from build123d import *

# Parameters (mm, degrees)
BASE_DEPTH                                          = 5
BASE_FILLET_R                                       = 1.65
HOOK_BASE_REACH                                     = 15.601
HOOK_BASE_END_RADIUS                                = 1.65
CBORE_FOR_M2_HEX_SOCKET_HEAD_CAP_SCREW1_D           = 2.4
CBORE_FOR_M2_HEX_SOCKET_HEAD_CAP_SCREW1_DEPTH       = 7.25
CBORE_FOR_M2_HEX_SOCKET_HEAD_CAP_SCREW1_CBORE_D     = 4.4
CBORE_FOR_M2_HEX_SOCKET_HEAD_CAP_SCREW1_CBORE_DEPTH = 2.4
CBORE_FOR_M2_HEX_SOCKET_HEAD_CAP_SCREW1_TIP         = 0.7210327428330723
SKETCH16_W                                          = 5.000000000000002
SKETCH16_H                                          = 1.65
SKETCH6_W                                           = 1.1499999999999981
SKETCH6_H                                           = 2.0000000000000004
CUT_EXTRUDE4_DEPTH                                  = 7.85
CIRPATTERN1_COUNT                                   = 2
FILLET1_R                                           = 1.65


with BuildPart() as part:
    # Sketch1 → Base (new body)
    # profile 1 of 2: a face of its own
    with BuildSketch(Plane(origin=(0, 0, 0), x_dir=(0, 1, 0), z_dir=(0, 0, 1))):
        Polygon((12.000000000000002, 4), (12.000000000000004, -3.9999999999999947), (-12, -4), (-12.000000000000002, 4), align=None)
        Polygon((-10, 2.35), (10, 2.35), (10, -2.35), (-9.999999999999998, -2.35), align=None, mode=Mode.SUBTRACT)
    # profile 2 of 2: a face of its own
    with BuildSketch(Plane(origin=(0, 0, 0), x_dir=(0, 1, 0), z_dir=(0, 0, 1))):
        Polygon((10, 2.35), (10, -2.35), (-9.999999999999998, -2.35), (-10, 2.35), align=None)
    extrude(amount=BASE_DEPTH)

    # Base-Fillet
    base_fillet_edges = [part.edges().sort_by_distance(p)[0] for p in [
        (-4, 0, 5),
        (3.9999999999999973, 1.78e-15, 5),
    ]]
    fillet(base_fillet_edges, radius=BASE_FILLET_R)

    # Hook Base: up to this cylinder (the profile starts outside it)
    hook_base_end = Plane(origin=(-2.35, 9.5, 3.35), z_dir=(0, 1, 0)) * Cylinder(HOOK_BASE_END_RADIUS, 35.502, mode=Mode.PRIVATE)
    # Sketch - Hook Base → Hook Base (add, up to the surface)
    with BuildSketch(Plane.XY.offset(5), mode=Mode.PRIVATE) as hook_base_sk1:
        Polygon((-4, 12.000000000000002), (-2.850000000000002, 12.000000000000004), (-2.850000000000002, 7.000000000000002), (-3.9999999999999982, 7.000000000000002), align=None)
    hook_base_tool1 = extrude(hook_base_sk1.sketch, amount=-HOOK_BASE_REACH, mode=Mode.PRIVATE) - hook_base_end
    hook_base = hook_base_tool1.solids().sort_by_distance((-3.425, 9.5, 5))[0]
    add(hook_base)

    # Hook: sweep along a path in Hook Path
    with BuildLine(Plane(origin=(-2.6e-15, 12.000000000000004, 0), x_dir=(-1, -2.2e-16, 0), z_dir=(-2.2e-16, 1, 0))) as hook_path:
        Line((2.849999999999999, 5.000000000000002), (2.85, 7.850000000000001))
        ThreePointArc((2.85, 7.850000000000001), (0.5876262664606571, 10.638762336766174), (-2.6076809620810604, 9.000000000000002))
    # Sketch - Hook Base<3> → Hook (sweep)
    with BuildSketch(Plane.XY.offset(5)):
        Polygon((-4, 12.000000000000002), (-2.850000000000002, 12.000000000000004), (-2.850000000000002, 7.000000000000002), (-3.9999999999999982, 7.000000000000002), align=None)
    hook = sweep(path=hook_path.line)

    # CBORE for M2 Hex Socket Head Cap Screw1
    with Locations(Plane(origin=(0, 0, 5), x_dir=(0, -1, 0), z_dir=(0, 0, 1))):
        with Locations((3.5, 0), (-3.5, 0)):
            CounterBoreHole(CBORE_FOR_M2_HEX_SOCKET_HEAD_CAP_SCREW1_D / 2, CBORE_FOR_M2_HEX_SOCKET_HEAD_CAP_SCREW1_CBORE_D / 2, CBORE_FOR_M2_HEX_SOCKET_HEAD_CAP_SCREW1_CBORE_DEPTH, depth=CBORE_FOR_M2_HEX_SOCKET_HEAD_CAP_SCREW1_DEPTH)
            with Locations((0, 0, -(CBORE_FOR_M2_HEX_SOCKET_HEAD_CAP_SCREW1_DEPTH + CBORE_FOR_M2_HEX_SOCKET_HEAD_CAP_SCREW1_TIP / 2))):  # 118° drill point
                Cone(0, CBORE_FOR_M2_HEX_SOCKET_HEAD_CAP_SCREW1_D / 2, CBORE_FOR_M2_HEX_SOCKET_HEAD_CAP_SCREW1_TIP, mode=Mode.SUBTRACT)

    # Sweep1: sweep along a path in Sketch15
    with BuildLine(Plane(origin=(-2.6e-15, 12.000000000000004, 0), x_dir=(-1, -2.2e-16, 0), z_dir=(-2.2e-16, 1, 0))) as sweep1_path:
        ThreePointArc((-8.7e-16, 5), (2.0152543263816596, 5.83474567361834), (2.849999999999999, 7.85))
    # Sketch16 → Sweep1 (sweep)
    with BuildSketch(Plane.YZ):
        with Locations((9.500000000000004, 4.175)):
            Rectangle(SKETCH16_W, SKETCH16_H)
    sweep1 = sweep(path=sweep1_path.line)

    # Sweep - Hook Rib: sweep along a path in Sketch8
    with BuildLine(Plane.YZ.offset(-3.425000000000001)) as sweep_hook_rib_path:
        Line((7.000000000000002, 5.3500000000000005), (4.999999999999995, 3.35))
    # Sketch6 → Sweep - Hook Rib (sweep)
    with BuildSketch(Plane.XZ.offset(-7.000000000000002)):
        with Locations((-3.4250000000000007, 4.3500000000000005)):
            Rectangle(SKETCH6_W, SKETCH6_H)
    sweep_hook_rib = sweep(path=sweep_hook_rib_path.line)

    # Sketch19 → Cut-Extrude4 (cut)
    with BuildSketch(Plane.XY.offset(7.85)):
        Polygon((-3.999999999999999, 7.000000000000002), (-3.999999999999999, 12.000000000000004), (-4.500000000000001, 12.000000000000002), (-4.499999999999999, 7.000000000000001), align=None)
    cut_extrude4 = extrude(amount=-CUT_EXTRUDE4_DEPTH, mode=Mode.SUBTRACT)

    # CirPattern1: Hook Base, Hook, Sweep1, Sweep - Hook Rib, Cut-Extrude4 ×2 about axis
    cirpattern1_axis = Axis((-6e-16, 1.16e-15, 0), (0, 0, 1))
    add([hook_base.rotate(cirpattern1_axis, i * 360 / CIRPATTERN1_COUNT) for i in range(1, CIRPATTERN1_COUNT)])
    add([hook.rotate(cirpattern1_axis, i * 360 / CIRPATTERN1_COUNT) for i in range(1, CIRPATTERN1_COUNT)])
    add([sweep1.rotate(cirpattern1_axis, i * 360 / CIRPATTERN1_COUNT) for i in range(1, CIRPATTERN1_COUNT)])
    add([sweep_hook_rib.rotate(cirpattern1_axis, i * 360 / CIRPATTERN1_COUNT) for i in range(1, CIRPATTERN1_COUNT)])
    add([cut_extrude4.rotate(cirpattern1_axis, i * 360 / CIRPATTERN1_COUNT) for i in range(1, CIRPATTERN1_COUNT)], mode=Mode.SUBTRACT)

    # Fillet1
    # the kernel refuses this fillet: 1.65 mm, written as the material it takes off along each edge
    with BuildSketch(Plane(origin=(-3.999999999999999, -12.000000000000002, -4.125000000000005), x_dir=(1, 0, 0), z_dir=(0, 0, 1))) as fillet1_piece_1:
        with BuildLine():
            CenterArc((FILLET1_R, FILLET1_R), FILLET1_R, 179.99999999999994, 90.00000000000006)
            Line((0, FILLET1_R), (0, 0))
            Line((0, 0), (FILLET1_R, 0))
        make_face()
    extrude(amount=7.475000000000006, mode=Mode.SUBTRACT)
    with BuildSketch(Plane(origin=(3.7e-16, -12.000000000000002, 7.850000000000004), x_dir=(-0.5093397654793319, 0, -0.8605655136603251), z_dir=(0.8605655136603251, 0, -0.5093397654793319))) as fillet1_piece_2:
        with BuildLine():
            CenterArc((2.8500000000000036 + FILLET1_R, FILLET1_R), FILLET1_R, 180, 90)
            Line((2.8500000000000036, FILLET1_R), (2.8500000000000036, 0))
            Line((2.8500000000000036, 0), (2.8500000000000036 + FILLET1_R, 0))
        make_face()
    revolve(axis=Axis((3.7e-16, -12.000000000000002, 7.850000000000004), (0, 1, 0)), revolution_arc=329.3801381453189, mode=Mode.SUBTRACT)
    with BuildSketch(Plane(origin=(3.9999999999999947, 12.000000000000004, -4.125000000000001), x_dir=(-1, 0, 0), z_dir=(0, 0, 1))) as fillet1_piece_3:
        with BuildLine():
            CenterArc((FILLET1_R, FILLET1_R), FILLET1_R, 180, 90)
            Line((-8.9e-16, FILLET1_R), (0, 0))
            Line((0, 0), (FILLET1_R, 0))
        make_face()
    extrude(amount=7.475000000000001, mode=Mode.SUBTRACT)
    with BuildSketch(Plane(origin=(3.9999999999999987, -12, 7.85), x_dir=(5.4e-16, 1, 0), z_dir=(-6e-17, 0, -1))) as fillet1_piece_4:
        with BuildLine():
            CenterArc((FILLET1_R, -FILLET1_R), FILLET1_R, 89.99999999999997, 90.00000000000003)
            Line((8.9e-16, -FILLET1_R), (0, 0))
            Line((0, 0), (FILLET1_R, 0))
        make_face()
    extrude(amount=11.975000000000005, mode=Mode.SUBTRACT)
    with BuildSketch(Plane(origin=(-2.66e-15, -12.000000000000002, 5), x_dir=(0, 0, -1), z_dir=(-1, -2.2e-16, 0))) as fillet1_piece_5:
        with BuildLine():
            CenterArc((FILLET1_R, -FILLET1_R), FILLET1_R, 90, 90)
            Line((0, -FILLET1_R), (0, 0))
            Line((0, 0), (FILLET1_R, 0))
        make_face()
    extrude(amount=2.349999999999998, mode=Mode.SUBTRACT)
    with BuildSketch(Plane(origin=(-3.05e-15, 12.000000000000004, 7.850000000000004), x_dir=(0.5093397654793319, 0, -0.8605655136603251), z_dir=(-0.8605655136603251, 0, -0.5093397654793319))) as fillet1_piece_6:
        with BuildLine():
            CenterArc((2.8500000000000036 + FILLET1_R, FILLET1_R), FILLET1_R, 180, 90)
            Line((2.8500000000000036, FILLET1_R), (2.8500000000000036, 0))
            Line((2.8500000000000036, 0), (2.8500000000000036 + FILLET1_R, 0))
        make_face()
    revolve(axis=Axis((-3.05e-15, 12.000000000000004, 7.850000000000004), (0, -1, 0)), revolution_arc=329.3801381453189, mode=Mode.SUBTRACT)
    with BuildSketch(Plane(origin=(8.125, -11.999999999999998, 0), x_dir=(0, 0, 1), z_dir=(-1, -2.2e-16, 0))) as fillet1_piece_7:
        with BuildLine():
            CenterArc((FILLET1_R, FILLET1_R), FILLET1_R, 180, 90)
            Line((-2.2e-16, FILLET1_R), (0, 0))
            Line((0, 0), (FILLET1_R, 0))
        make_face()
    extrude(amount=16.25, mode=Mode.SUBTRACT)
    with BuildSketch(Plane(origin=(-8.125, 12, 0), x_dir=(0, 0, 1), z_dir=(1, 2.2e-16, 0))) as fillet1_piece_8:
        with BuildLine():
            CenterArc((FILLET1_R, FILLET1_R), FILLET1_R, 180, 90)
            Line((-2.2e-16, FILLET1_R), (0, 0))
            Line((0, 0), (FILLET1_R, 0))
        make_face()
    extrude(amount=16.249999999999993, mode=Mode.SUBTRACT)
    with BuildSketch(Plane(origin=(0, 12.000000000000004, 5), x_dir=(0, 0, -1), z_dir=(1, 2.2e-16, 0))) as fillet1_piece_9:
        with BuildLine():
            CenterArc((FILLET1_R, -FILLET1_R), FILLET1_R, 90, 90)
            Line((0, -FILLET1_R), (0, 0))
            Line((0, 0), (FILLET1_R, 0))
        make_face()
    extrude(amount=2.349999999999995, mode=Mode.SUBTRACT)
    with BuildSketch(Plane(origin=(-3.999999999999999, 12.000000000000002, -4.124999999999998), x_dir=(1, 0, 2.3e-16), z_dir=(-2.3e-16, -4.5e-16, 1))) as fillet1_piece_10:
        with BuildLine():
            CenterArc((FILLET1_R, -FILLET1_R), FILLET1_R, 90.00000000000001, 89.99999999999999)
            Line((0, -FILLET1_R), (0, 0))
            Line((0, 0), (FILLET1_R, 0))
        make_face()
    extrude(amount=11.974999999999998, mode=Mode.SUBTRACT)
    with BuildSketch(Plane(origin=(3.7e-16, -12, 7.850000000000004), x_dir=(1, 0, -1.33e-15), z_dir=(-1.33e-15, 0, -1))) as fillet1_piece_11:
        with BuildLine():
            CenterArc((3.9999999999999982 - FILLET1_R, -FILLET1_R), FILLET1_R, 6.168e-14, 89.99999999999994)
            Line((3.9999999999999982, -FILLET1_R), (3.9999999999999982, 0))
            Line((3.9999999999999982, 0), (3.9999999999999982 - FILLET1_R, 0))
        make_face()
    revolve(axis=Axis((3.7e-16, -12, 7.850000000000004), (-1.2e-16, -1, 0)), revolution_arc=215.36009714129503, mode=Mode.SUBTRACT)
    with BuildSketch(Plane(origin=(2.349999999999995, 12.000000000000004, 3.3500000000000005), x_dir=(1, 0, 0), z_dir=(0, 0, -1))) as fillet1_piece_12:
        with BuildLine():
            CenterArc((1.65 - FILLET1_R, FILLET1_R), FILLET1_R, 270, 90.00000000000001)
            Line((1.6500000000000004, FILLET1_R), (1.65, 0))
            Line((1.65, 0), (1.65 - FILLET1_R, 0))
        make_face()
    revolve(axis=Axis((2.349999999999995, 12.000000000000004, 3.3500000000000005), (2.2e-16, -1, 0)), revolution_arc=90, mode=Mode.SUBTRACT)
    with BuildSketch(Plane(origin=(-2.3500000000000005, -12, 3.3500000000000005), x_dir=(-1, 0, -2.7e-16), z_dir=(2.7e-16, 0, -1))) as fillet1_piece_13:
        with BuildLine():
            CenterArc((1.6499999999999995 - FILLET1_R, FILLET1_R), FILLET1_R, 270, 90.00000000000007)
            Line((1.6499999999999995, FILLET1_R), (1.6499999999999995, 0))
            Line((1.6499999999999995, 0), (1.6499999999999995 - FILLET1_R, -1.78e-15))
        make_face()
    revolve(axis=Axis((-2.3500000000000005, -12, 3.3500000000000005), (0, 1, 0)), revolution_arc=90, mode=Mode.SUBTRACT)
    with BuildSketch(Plane(origin=(-3.05e-15, 12.000000000000002, 7.850000000000004), x_dir=(-1, 0, -1.33e-15), z_dir=(1.33e-15, 0, -1))) as fillet1_piece_14:
        with BuildLine():
            CenterArc((3.9999999999999987 - FILLET1_R, -FILLET1_R), FILLET1_R, 0, 90)
            Line((3.9999999999999987, -FILLET1_R), (3.9999999999999987, 0))
            Line((3.9999999999999987, 0), (3.9999999999999987 - FILLET1_R, 0))
        make_face()
    revolve(axis=Axis((-3.05e-15, 12.000000000000002, 7.850000000000004), (0, 1, 0)), revolution_arc=215.36009714129503, mode=Mode.SUBTRACT)


solid = part.part
Read the model definition and answer for the solid it produces. Units are mm, in the model's axes. A direction names the side the tool comes from. Coordinates: 2 decimals unless noted, no trailing zeros. Loops run counter-clockwise (first coordinate to the right, second up) from the corner with the lowest first, then second, coordinate; pieces in that order, holes last. Notation, with made-up numbers: (80, 42) - (136, 42) arc R12 cw to (136, 60) - close; hole circle Ø1 at (37, -5). An arc over 180 degrees is marked (long way). Answer in a Markdown table with one row per item.
Q1. Find section B-B on z = 3. Write down the section's boundary in (x, y).
Here are the results:
| item | result |
|---|---|
| outline | (-4, -10.35) arc R1.65 ccw to (-2.35, -12) - (2.35, -12) arc R1.65 ccw to (4, -10.35) - (4, 10.35) arc R1.65 ccw to (2.35, 12) - (-2.35, 12) arc R1.65 ccw to (-4, 10.35) - close; hole circle Ø4.4 at (0, -3.5); hole circle Ø4.4 at (0, 3.5) |
Q2. Find section C-C on y = -7.75. Write down the section's boundary in (x, z), plus the area to 3 significant figures.
Here are the results:
| item | result |
|---|---|
| outline | (-4, 0) - (4, 0) - (4, 7.85) arc R4 ccw to (-3.66, 9.46) - (-2.61, 9) arc R2.85 cw (long way) to (0, 5) - (-2.35, 5) arc R1.65 ccw to (-4, 3.35) - close |
| area | 55.2 mm^2 |
Q3. Straight lines are drawn through the part: line 1 along Y through (x, z) = (1, 1.25); line 2 along Y through (x, z) = (1.5, 3); line 3 along Z through (x, y) = (0, 7.95). For each, find the intervals that lie inside material, in ascending order. Write a range as [from, to].
Here are the results:
| item | result |
|---|---|
| line 1 | y = [-11.95, -4.16], [-2.84, 2.84], [4.16, 11.95] |
| line 2 | y = [-12, -5.11], [-1.89, 1.89], [5.11, 12] |
| line 3 | z = [0, 5], [10.7, 11.85] |
Q4. Find section A-A on y = 3.5. Write down the section's boundary in (x, z).
Here are the results:
| item | result |
|---|---|
| outline | (-4, 0) - (-1.2, 0) - (-1.2, 2.6) - (-2.2, 2.6) - (-2.2, 5) - (-2.35, 5) arc R1.65 ccw to (-4, 3.35) - close; (1.2, 0) - (4, 0) - (4, 3.35) arc R1.65 ccw to (2.35, 5) - (2.2, 5) - (2.2, 2.6) - (1.2, 2.6) - close |
Q5. The mould has two halves that part along Y. Classify faces 1 (the cylindrical face through (2.433, -8.652, 9.334)), 2 (the flat face through (-1.9, 7, 10.2)), 3 (the flat face through (-1.4, 3.5, 2.6)), 4 (the flat face through (0, 12, 3)): pulls with the +Y half, pulls with the -Y half, needs draft (parallel to the pull), parting line crosses it, or undercut.
Here are the results:
| item | result |
|---|---|
| face 1 | needs draft |
| face 2 | undercut |
| face 3 | undercut |
| face 4 | pulls with the +Y half |
Q6. Given P1, Ø1.3, axis at x = 0, y = -4.5, coming from the +Z side; P2, Ø3, axis at x = 0.5, y = -5, coming from the -Z side; P3, Ø3.5, axis at x = 0, z = 7.85, coming from the +Y side; P4, Ø0.5, axis at y = 7, z = 5, coming from the +X side, each flat-ended and moving along its own axis, determine where each tip first touches the part or whether it passes through.
Here are the results:
| item | result |
|---|---|
| P1 | stops at z = 2.6 |
| P2 | stops at z = 0 |
| P3 | passes through |
| P4 | stops at x = 3.22 |
Q7. For faces 5 (the flat face through (3.54, -6.43, 4.78)), 6 (the flat face through (-1.4, -3.5, 2.6)), 7 (the cylindrical face through (1.159, 11.529, 4.504)), determine the directions among +Z, -Z, +X, -X, +Y, -Y from which every point of the face is accessible in a straight line to the end or side of a thin tool.
Here are the results:
| item | result |
|---|---|
| face 5 | +Z, +X, +Y |
| face 6 | +Z |
| face 7 | +X, +Y |
Q8. Find section D-D on y = -3.25. Write down the section's boundary in (x, z).
Here are the results:
| item | result |
|---|---|
| outline | (-4, 0) - (-1.17, 0) - (-1.17, 2.6) - (-2.19, 2.6) - (-2.19, 5) - (-2.35, 5) arc R1.65 ccw to (-4, 3.35) - close; (1.17, 0) - (4, 0) - (4, 3.35) arc R1.65 ccw to (2.35, 5) - (2.19, 5) - (2.19, 2.6) - (1.17, 2.6) - close |
